Verification items for this drawing (mm, ordinates from the low corner). Coordinates: 2 decimals unless noted, no trailing zeros. Write each loop counter-clockwise with the first axis right and the second up, starting at its lowest first coordinate (ties: lowest second). Pieces come first, ordered by that corner, then holes. Notation, with made-up numbers: (6.25, 15.5) -> (47.25, 15.5) arc R13 ccw to (47.25, 24.5) -> close; hole circle Ø11 at (7, -21). An arc over 180 degrees is marked (long way). One line per question, with ' | ' between items.
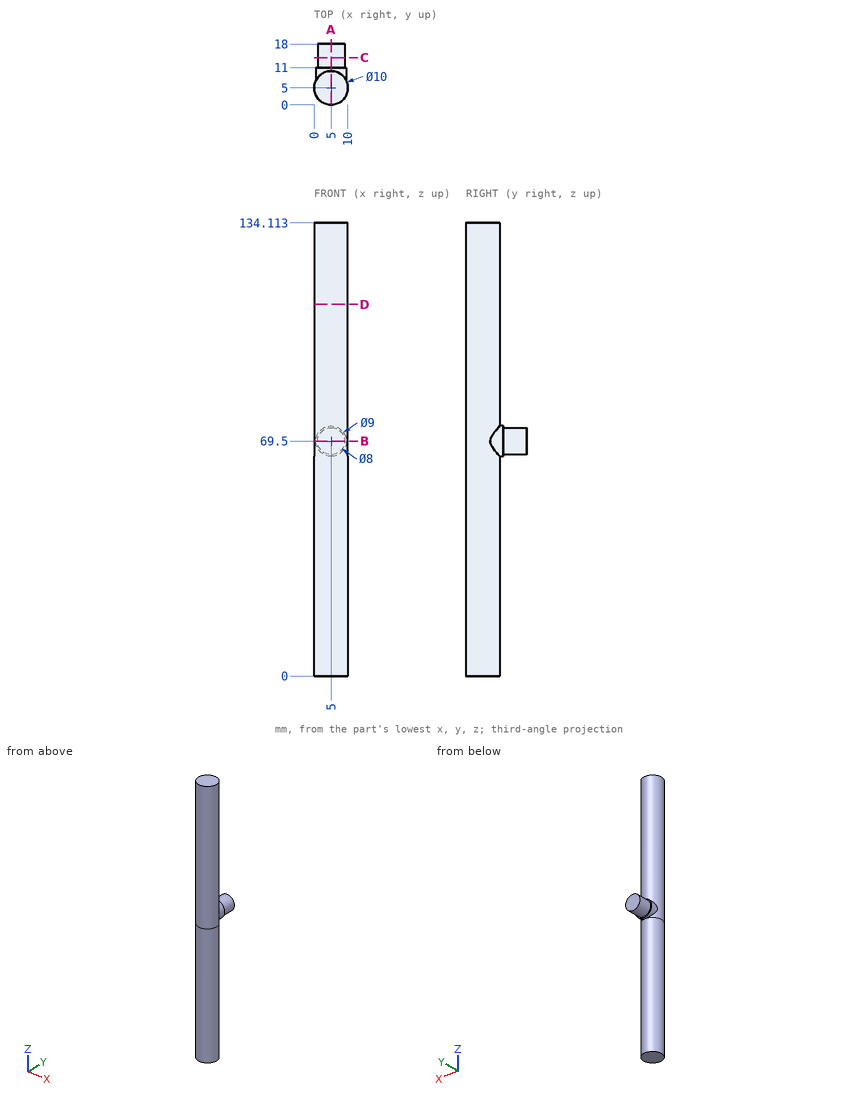
(1) Cross-section at A-A (x = 5). Record the cut outline in (y, z).
Answers below:
outline: (0, 0) -> (10, 0) -> (10, 65) -> (11, 65) -> (11, 65.5) -> (18, 65.5) -> (18, 73.5) -> (11, 73.5) -> (11, 74) -> (10, 74) -> (10, 134.11) -> (0, 134.11) -> close
(2) Cross-section at D-D (z = 110). Record the cut outline in (x, y).
Answers below:
outline: circle Ø10 at (5, 5)
(3) Cross-section at B-B (z = 69.5). Record the cut outline in (x, y).
Answers below:
outline: (0.5, 7.18) arc R5 ccw (long way) to (9.5, 7.18) -> (9.5, 11) -> (9, 11) -> (9, 18) -> (1, 18) -> (1, 11) -> (0.5, 11) -> close
(4) Depth check by flat-ended pin: P1, Ø2, axis at x = 3.5, z = 96, coming from the +Y side (1 decimal); P2, Ø1.5, axis at x = 8.5, z = 114, coming from the -Y side (1 decimal); P3, Ø3, axis at x = 7, z = 36, coming from the -Y side (1 decimal). Enter the tip coordinate at first touch or a pass-through.
Answers below:
P1: stops at y = 10 | P2: stops at y = 0.8 | P3: stops at y = 0
(5) Cross-section at C-C (y = 14). Record the cut outline in (x, z).
Answers below:
outline: circle Ø8 at (5, 69.5)
(6) Material ranges on line 1 (X direction, y = 2, z = 50); line 2 (Y direction, x = 5, z = 64.5), recorded low to high.
Answers below:
line 1: x = 1 to 9 | line 2: y = 0 to 10
